from build123d import *

# Parameters (mm, degrees)
BASES_W                = 27
BASES_H                = 18
BASE_DEPTH             = 6.5
DIAMONDCUT_DEPTH       = 5
O_RINGPROFILE_DEPTH    = 1.3
SPRINGRETENTIONS_W     = 0.95
SPRINGRETENTIONS_H     = 2.5
M3_CLEARANCE_HOLE1_D   = 3.5
MOUNTINGHOLECUTS_DEPTH = 3.5
BASEF_R                = 0.5


with BuildPart() as part:
    # BaseS → Base (new body)
    with BuildSketch(Plane(origin=(0, 0, 0), x_dir=(1, 0, 0), z_dir=(0, 1, 0))):
        Rectangle(BASES_W, BASES_H)
    extrude(amount=BASE_DEPTH)

    # DiamondCutS → DiamondCut (cut)
    with BuildSketch(Plane(origin=(0, 6.5, 0), x_dir=(1, 0, 0), z_dir=(0, 1, 0))):
        with BuildLine():
            Line((-1.566008472, 3.61128036), (8.554644537, 5.984544502))
            ThreePointArc((8.554644537, 5.984544502), (8.81973312, 5.87982208), (8.814442824, 5.594847071))
            Line((8.814442824, 5.594847071), (2.731178612, -2.834500266))
            ThreePointArc((2.731178612, -2.834500266), (2.218800785, -3.328201177), (1.566008472, -3.61128036))
            Line((1.566008472, -3.61128036), (-8.554644537, -5.984544502))
            ThreePointArc((-8.554644537, -5.984544502), (-8.81973312, -5.87982208), (-8.814442824, -5.594847071))
            Line((-8.814442824, -5.594847071), (-2.731178612, 2.834500266))
            ThreePointArc((-2.731178612, 2.834500266), (-2.218800785, 3.328201177), (-1.566008472, 3.61128036))
        make_face()
    extrude(amount=-DIAMONDCUT_DEPTH, mode=Mode.SUBTRACT)

    # O-RingProfileS → O-RingProfile (cut)
    with BuildSketch(Plane(origin=(0, 6.5, 0), x_dir=(1, 0, 0), z_dir=(0, 1, 0))):
        with BuildLine():
            Line((4.677312477, -4.238979879), (10.760576688, 4.190367458))
            ThreePointArc((10.760576688, 4.190367458), (10.816653826, 7.211102551), (8.006714841, 8.321160228))
            Line((8.006714841, 8.321160228), (-2.113938167, 5.947896086))
            ThreePointArc((-2.113938167, 5.947896086), (-3.550081256, 5.325121884), (-4.677312477, 4.238979879))
            Line((-4.677312477, 4.238979879), (-10.760576688, -4.190367458))
            ThreePointArc((-10.760576688, -4.190367458), (-10.816653826, -7.211102551), (-8.006714841, -8.321160228))
            Line((-8.006714841, -8.321160228), (2.113938167, -5.947896086))
            ThreePointArc((2.113938167, -5.947896086), (3.550081256, -5.325121884), (4.677312477, -4.238979879))
        make_face()
        with BuildLine():
            Line((3.379889901, -3.302660137), (9.463154112, 5.1266872))
            ThreePointArc((9.463154112, 5.1266872), (9.485373355, 6.323582237), (8.372001305, 6.763416411))
            Line((8.372001305, 6.763416411), (-1.748651703, 4.390152269))
            ThreePointArc((-1.748651703, 4.390152269), (-2.662560942, 3.993841413), (-3.379889901, 3.302660137))
            Line((-3.379889901, 3.302660137), (-9.463154112, -5.1266872))
            ThreePointArc((-9.463154112, -5.1266872), (-9.485373355, -6.323582237), (-8.372001305, -6.763416411))
            Line((-8.372001305, -6.763416411), (1.748651703, -4.390152269))
            ThreePointArc((1.748651703, -4.390152269), (2.662560942, -3.993841413), (3.379889901, -3.302660137))
        make_face(mode=Mode.SUBTRACT)
    extrude(amount=-O_RINGPROFILE_DEPTH, mode=Mode.SUBTRACT)

    # SpringRetentionS → SpringRetention (revolve)
    with BuildSketch(Plane(origin=(0, 0, 0), x_dir=(0, 0, -1), z_dir=(1, 0, 0))):
        with Locations((0.475, 2.75)):
            Rectangle(SPRINGRETENTIONS_W, SPRINGRETENTIONS_H)
    revolve(axis=Axis((0, 1.5, 0), (0, 1, 0)))

    # M3 Clearance Hole1 (through all)
    with Locations(Plane(origin=(0, 6.5, 0), x_dir=(-1, 0, 0), z_dir=(0, 1, 0))):
        with Locations((10, -5), (-10, 5)):
            Hole(M3_CLEARANCE_HOLE1_D / 2)

    # MountingHoleCutsS → MountingHoleCuts (cut)
    with BuildSketch(Plane.XZ):
        with BuildLine():
            Line((13.5, 1.5), (13.5, 9))
            Line((13.5, 9), (6, 9))
            Line((6, 9), (6, 6))
            ThreePointArc((6, 6), (7.318019485, 2.818019485), (10.5, 1.5))
            Line((10.5, 1.5), (13.5, 1.5))
        make_face()
        with BuildLine():
            Line((-13.5, -9), (-6, -9))
            Line((-6, -9), (-6, -6))
            ThreePointArc((-6, -6), (-7.318019485, -2.818019485), (-10.5, -1.5))
            Line((-10.5, -1.5), (-13.5, -1.5))
            Line((-13.5, -1.5), (-13.5, -9))
        make_face()
    extrude(amount=-MOUNTINGHOLECUTS_DEPTH, mode=Mode.SUBTRACT)

    # BaseF
    basef_edges = [part.edges().sort_by_distance(p)[0] for p in [
        (-6, 1.75, -9),
        (-13.5, 1.75, -1.5),
        (6, 1.75, 9),
        (13.5, 1.75, 1.5),
        (13.5, 5, 9),
        (-13.5, 3.25, 9),
        (-13.5, 5, -9),
        (13.5, 3.25, -9),
    ]]
    fillet(basef_edges, radius=BASEF_R)


solid = part.part
Could you check a few things on this model? Use its own coordinates, in mm. A direction names the side the tool comes from. Coordinates: 2 decimals unless noted, no trailing zeros. Order: outer loops, then holes, each group sorted by start corner. A loop starts at its lowest first (then second) coordinate and runs counter-clockwise, first axis right, second up.
Q1. Suppose I cut it at B-B on x = 10. Please give me the cut outline in (y, z).
Q2. Suppose I cut it at A-A on y = 2. Please give me the cut outline in (x, z), and give its area (3 significant figures).
Q3. Please list where these lines run through material, in increasing order: L1, parallel to Z at x = 10, y = 4.9; L2, parallel to Z at x = 10, y = 5.6; L3, parallel to Z at x = -10, y = 5.1.
Q4. Suppose I cut it at C-C on x = 0. Please give me the cut outline in (y, z), and give its area (3 significant figures).
Q5. Thinking about a two-plate mould opening in Z: for faces 4 (the cylindrical face through (7.283, 1.726, 2.853)), 5 (the cylindrical face through (3.53, 5.86, 5.34)), 6 (the flat face through (6, 2, 7)), which applies, released by +Z, released by -Z, zero draft, split by the parting line, or undercut?
Q6. Which directions (+Z, -Z, +X, -X, +Y, -Y) give clear straight access to the entire face, cutting with the end or side of a thin tool? Please do faces 1 (the flat face through (3, 3, -9)), 2 (the flat face through (-12, 2, -1.5)), 3 (the flat face through (5.815, 4.035, -1.439)).
Q7. Will these pins go through, and if not, where does the flat tip stop? pin 1 (1.2 mm diameter, centred on x = -11.5, y = 2.5, fed in from -Z); pin 2 (5.5 mm diameter, centred on x = -10, z = -5, fed in from -Y); pin 3 (1.2 mm diameter, centred on y = 2, z = -7.5, fed in from -X).
Q8. Suppose I cut it at D-D on z = 0. Please give me the cut outline in (x, y), and give its area (3 significant figures).
Answer:
1. outline: (0, -9) - (6.5, -9) - (6.5, -8) - (5.2, -8) - (5.2, -3.14) - (6.5, -3.14) - (6.5, 3.25) - (3.5, 3.25) - (3.5, 1.53) - (0, 1.53) - close; (3.5, 6.75) - (6.5, 6.75) - (6.5, 9) - (3.5, 9) - close
2. outline: (-13.5, -1) arc R0.5 ccw to (-13, -1.5) - (-10.5, -1.5) arc R4.5 cw to (-6, -6) - (-6, -8.5) arc R0.5 ccw to (-5.5, -9) - (13, -9) arc R0.5 ccw to (13.5, -8.5) - (13.5, 1) arc R0.5 ccw to (13, 1.5) - (10.5, 1.5) arc R4.5 cw to (6, 6) - (6, 8.5) arc R0.5 ccw to (5.5, 9) - (-13, 9) arc R0.5 ccw to (-13.5, 8.5) - close; circle Ø1.9 at (0, 0); hole (-8.81, 5.59) - (-2.73, -2.83) arc R2 ccw to (-1.57, -3.61) - (8.55, -5.98) arc R0.25 ccw to (8.81, -5.59) - (2.73, 2.83) arc R2 ccw to (1.57, 3.61) - (-8.55, 5.98) arc R0.25 ccw to start
2. area: 294 mm2
3. L1: z = -9 to 3.25, 6.75 to 9
3. L2: z = -9 to -8, -3.14 to 3.25, 6.75 to 9
3. L3: z = -9 to -6.75, -3.25 to 9
4. outline: (0, -9) - (6.5, -9) - (6.5, -6.44) - (5.2, -6.44) - (5.2, -4.8) - (6.5, -4.8) - (6.5, -3.98) - (1.5, -3.98) - (1.5, -0.95) - (4, -0.95) - (4, 0.95) - (1.5, 0.95) - (1.5, 3.98) - (6.5, 3.98) - (6.5, 4.8) - (5.2, 4.8) - (5.2, 6.44) - (6.5, 6.44) - (6.5, 9) - (0, 9) - close
4. area: 77.7 mm2
5. face 4: released by +Z
5. face 5: undercut
5. face 6: zero draft
6. face 1: -Z, +X, -X, +Y, -Y
6. face 2: -Z, -X, -Y
6. face 3: +Y
7. pin 1: stops at z = -1.5
7. pin 2: stops at y = 3.5
7. pin 3: stops at x = -6
8. outline: (-13.5, 0) - (13.5, 0) - (13.5, 6.5) - (7.74, 6.5) - (7.74, 5.2) - (5.76, 5.2) - (5.76, 6.5) - (4.78, 6.5) - (4.78, 1.5) - (0.95, 1.5) - (0.95, 4) - (-0.95, 4) - (-0.95, 1.5) - (-4.78, 1.5) - (-4.78, 6.5) - (-5.76, 6.5) - (-5.76, 5.2) - (-7.74, 5.2) - (-7.74, 6.5) - (-13.5, 6.5) - close
8. area: 127 mm2
